```python
from build123d import *

# Parameters (mm, degrees)
SKETCH1_R           = 8
BOSS_EXTRUDE1_DEPTH = 5


with BuildPart() as part:
    # Sketch1 → Boss-Extrude1 (new, symmetric)
    with BuildSketch(Plane.XY):
        Polygon((-20, -50), (20, -50), (20, 40), (10, 50), (-10, 50), (-20, 40), align=None)
        with Locations((0, 20)):
            Circle(SKETCH1_R, mode=Mode.SUBTRACT)
    extrude(amount=BOSS_EXTRUDE1_DEPTH, both=True)


solid = part.part
```
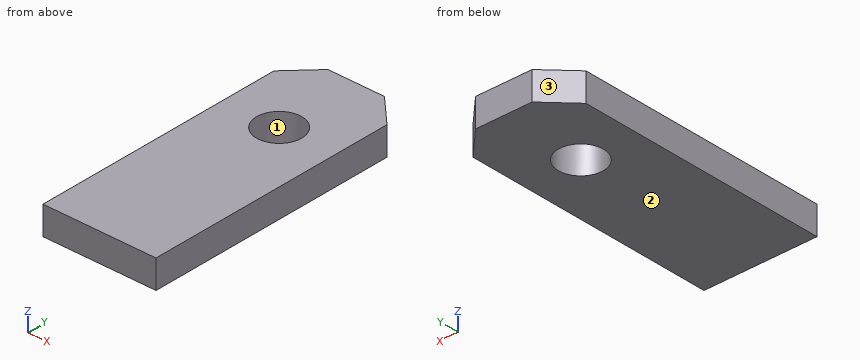
Here's how the part is built. I have some questions about the finished solid (model axes, mm). Face numbers are marked on the shaded views. Coordinates: 2 decimals unless noted, no trailing zeros. Write each loop counter-clockwise with the first axis right and the second up, starting at its lowest first coordinate (ties: lowest second). Pieces come first, ordered by that corner, then holes. Notation, with made-up numbers: M 26,-12.75 L 78,-12.75 A7 cw 78,-5.75 Z; hole C 56.25,-18.5 d3. An arc over 180 degrees is marked long. Answer as CSV lines item,"result". Start each with the question number.
Q1. Suppose I cut it at C-C, the plane y = 20. List the corners of the cut face in (x, z) for me.
Q2. I need wall thicknesses on probe 1 along Y at (x, z) = (0, 2.5); probe 2 along X at (y, z) = (18, 0.5); probe 3 along Y at (x, z) = (6, 3.25). Which ranges of each line are inside material? Lowest first, please. Write a range as [from, to].
Q3. Will these pins go through, and if not, where does the flat tip stop? pin 1 Ø1.5 at (x, z) = (14, -1.5) entering from +Y; pin 2 Ø14.5 at (x, y) = (0, 20) entering from +Z.
Q4. Suppose I cut it at A-A, the plane x = 0. List the corners of the cut face in (y, z) for me, then the cut area to 3 significant figures.
Q5. If we mould it in two halves opening along Y, with no side actions, what happens to the marked faces 1, 2 and 3? For each: pulls with the +Y half, pulls with the -Y half, needs draft (parallel to the pull), parting line crosses it, or undercut.
Q6. Suppose I cut it at D-D, the plane x = -16. List the corners of the cut face in (y, z) for me.
Q7. Suppose I cut it at B-B, the plane z = -1.25. List the corners of the cut face in (x, y) for me.
Entries:
1,outline,"M -20,-5 L -8,-5 L -8,5 L -20,5 Z; M 8,-5 L 20,-5 L 20,5 L 8,5 Z"
2,probe 1,"y = [-50, 12], [28, 50]"
2,probe 2,"x = [-20, -7.75], [7.75, 20]"
2,probe 3,"y = [-50, 14.71], [25.29, 50]"
3,pin 1,"stops at y = 46.75"
3,pin 2,"passes through"
4,outline,"M -50,-5 L 12,-5 L 12,5 L -50,5 Z; M 28,-5 L 50,-5 L 50,5 L 28,5 Z"
4,area,"840 mm²"
5,face 1,"undercut"
5,face 2,"needs draft"
5,face 3,"pulls with the +Y half"
6,outline,"M -50,-5 L 44,-5 L 44,5 L -50,5 Z"
7,outline,"M -20,-50 L 20,-50 L 20,40 L 10,50 L -10,50 L -20,40 Z; hole C 0,20 d16"
